CAD build for the part. Positions are in the model's coordinates, mm. A direction names the side the tool comes from. Give positions to 0.01 mm unless a question says otherwise; leave off trailing zeros. Order: outer loops, then holes, each group sorted by start corner. A loop starts at its lowest first (then second) coordinate and runs counter-clockwise, first axis right, second up. Notation, with made-up numbers: (83.5, -19) -> (119.5, -19) arc R28 ccw to (119.5, 3) -> close; hole circle Ø8 at (-10, 58). An arc over 180 degrees is marked (long way). Use one line per item in the form item = value. Start each with the question number.
1) Tool access for faces 1 (the face through (5, 1, 0)), 2 (the face through (2.7, 1.5, -2.948)): list every direction of +Z, -Z, +X, -X, +Y, -Y with a clear straight run to the whole face (end or side of a thin tool).
2) Probe line 1 (Z direction, x = 2.25, y = 0.3); line 2 (X direction, y = 1.3, z = -1.75); line 3 (Z direction, x = 1, y = 2.35). List the from-to ranges inside material, lowest first.
3) Cut at C-C, the plane z = -0.75. Give the cut face in (x, y).
4) Cut at A-A, the plane y = 0.7. Give the cut face in (x, z), and give its area (3 significant figures).
5) Mould opens along X. For faces 3 (the face through (0, 1, -4)), 4 (the face through (5, 1, -8)), 5 (the face through (1, 2, -0.5)), 6 (the face through (10, 1, -4)) say: pulls with the +X half, pulls with the -X half, needs draft (parallel to the pull), parting line crosses it, or undercut.
6) Cut at B-B, the plane x = 2.5. Give the cut face in (y, z).
from build123d import *

# Parameters (mm, degrees)
SKETCH1_W           = 10
SKETCH1_H           = 8
BOSS_EXTRUDE1_DEPTH = 3
CUT_EXTRUDE1_REACH  = 15.153


with BuildPart() as part:
    # Sketch1 → Boss-Extrude1 (new body)
    with BuildSketch(Plane(origin=(0, 0, 0), x_dir=(1, 0, 0), z_dir=(0, 1, 0))):
        with Locations((5, 4)):
            Rectangle(SKETCH1_W, SKETCH1_H)
    extrude(amount=BOSS_EXTRUDE1_DEPTH)

    # Sketch2 → Cut-Extrude1 (cut, up to next)
    with BuildSketch(Plane(origin=(0, 3, 0), x_dir=(1, 0, 0), z_dir=(0, 1, 0)), mode=Mode.PRIVATE) as cut_extrude1_sk1:
        Polygon((2.076794919, 1.291025404), (1.620096189, 2.082050808), (0.70669873, 2.082050808), (0.25, 1.291025404), (0.70669873, 0.5), (1.620096189, 0.5), align=None)
    cut_extrude1_tool1 = extrude(cut_extrude1_sk1.sketch, amount=-CUT_EXTRUDE1_REACH, mode=Mode.PRIVATE) & part.part
    # Sketch2 → Cut-Extrude1 (cut, up to next)
    with BuildSketch(Plane(origin=(0, 3, 0), x_dir=(1, 0, 0), z_dir=(0, 1, 0)), mode=Mode.PRIVATE) as cut_extrude1_sk2:
        Polygon((3.576794919, 2.157050808), (3.120096189, 2.948076211), (2.20669873, 2.948076211), (1.75, 2.157050808), (2.20669873, 1.366025404), (3.120096189, 1.366025404), align=None)
    cut_extrude1_tool2 = extrude(cut_extrude1_sk2.sketch, amount=-CUT_EXTRUDE1_REACH, mode=Mode.PRIVATE) & part.part
    add(cut_extrude1_tool1.solids().sort_by_distance((1.163397, 3, -1.291025))[0], mode=Mode.SUBTRACT)
    add(cut_extrude1_tool2.solids().sort_by_distance((2.663397, 3, -2.157051))[0], mode=Mode.SUBTRACT)


solid = part.part
Result:
q1.face_1 = +Z, +X, -X, +Y, -Y
q1.face_2 = +Y, -Y
q2.line_1 = -8 to -2.95, -1.37 to 0
q2.line_2 = 0 to 0.51, 1.81 to 1.99, 3.34 to 10
q2.line_3 = -8 to -2.08, -0.5 to 0
q3.outline = (0, 0) -> (0.56, 0) -> (0.56, 3) -> (0, 3) -> close; (1.76, 0) -> (10, 0) -> (10, 3) -> (1.76, 3) -> close
q4.outline = (0, -8) -> (10, -8) -> (10, 0) -> (0, 0) -> close; hole (0.25, -1.29) -> (0.71, -2.08) -> (1.62, -2.08) -> (2.08, -1.29) -> (1.62, -0.5) -> (0.71, -0.5) -> close; hole (1.75, -2.16) -> (2.21, -2.95) -> (3.12, -2.95) -> (3.58, -2.16) -> (3.12, -1.37) -> (2.21, -1.37) -> close
q4.area = 75.7 mm²
q5.face_3 = pulls with the -X half
q5.face_4 = needs draft
q5.face_5 = undercut
q5.face_6 = pulls with the +X half
q6.outline = (0, -8) -> (3, -8) -> (3, -2.95) -> (0, -2.95) -> close; (0, -1.37) -> (3, -1.37) -> (3, 0) -> (0, 0) -> close
